from build123d import *

# Parameters (mm, degrees)
SKETCH_1_W          = 9
SKETCH_1_H          = 6.5
EXTRUDE_1_DEPTH     = 815
SKETCH_2_R          = 1.750000006
CUT_EXTRUDE_1_DEPTH = 726.778225985
SKETCH_3_R          = 3.000000006
CUT_EXTRUDE_2_DEPTH = 3.5


with BuildPart() as part:
    # 草图1 → 凸台-拉伸1 (new body)
    with BuildSketch(Plane.XY.offset(-89.264832522)):
        Rectangle(SKETCH_1_W, SKETCH_1_H)
    extrude(amount=EXTRUDE_1_DEPTH)

    # 草图2 → 切除-拉伸1 (cut, through all)
    with BuildSketch(Plane(origin=(0, 3.25, 0), x_dir=(1, 0, 0), z_dir=(0, 1, 0))):
        with Locations(Location((0, 81.764832522, 0), (0, 0, 270))):
            Circle(SKETCH_2_R)
        with Locations(Location((0, 61.764832522, 0), (0, 0, 270))):
            Circle(SKETCH_2_R)
        with Locations(Location((0, 41.764832522, 0), (0, 0, 270))):
            Circle(SKETCH_2_R)
        with Locations(Location((0, 21.764832522, 0), (0, 0, 270))):
            Circle(SKETCH_2_R)
        with Locations(Location((0, 1.764832522, 0), (0, 0, 270))):
            Circle(SKETCH_2_R)
        with Locations(Location((0, -18.235167478, 0), (0, 0, 270))):
            Circle(SKETCH_2_R)
        with Locations(Location((0, -38.235167478, 0), (0, 0, 270))):
            Circle(SKETCH_2_R)
        with Locations(Location((0, -58.235167478, 0), (0, 0, 270))):
            Circle(SKETCH_2_R)
        with Locations(Location((0, -78.235167478, 0), (0, 0, 270))):
            Circle(SKETCH_2_R)
        with Locations(Location((0, -98.235167478, 0), (0, 0, 270))):
            Circle(SKETCH_2_R)
        with Locations(Location((0, -118.235167478, 0), (0, 0, 270))):
            Circle(SKETCH_2_R)
        with Locations(Location((0, -138.235167478, 0), (0, 0, 270))):
            Circle(SKETCH_2_R)
        with Locations(Location((0, -158.235167478, 0), (0, 0, 270))):
            Circle(SKETCH_2_R)
        with Locations(Location((0, -178.235167478, 0), (0, 0, 270))):
            Circle(SKETCH_2_R)
        with Locations(Location((0, -198.235167478, 0), (0, 0, 270))):
            Circle(SKETCH_2_R)
        with Locations(Location((0, -218.235167478, 0), (0, 0, 270))):
            Circle(SKETCH_2_R)
        with Locations(Location((0, -238.235167478, 0), (0, 0, 270))):
            Circle(SKETCH_2_R)
        with Locations(Location((0, -258.235167478, 0), (0, 0, 270))):
            Circle(SKETCH_2_R)
        with Locations(Location((0, -278.235167478, 0), (0, 0, 270))):
            Circle(SKETCH_2_R)
        with Locations(Location((0, -298.235167478, 0), (0, 0, 270))):
            Circle(SKETCH_2_R)
        with Locations(Location((0, -318.235167478, 0), (0, 0, 270))):
            Circle(SKETCH_2_R)
        with Locations(Location((0, -338.235167478, 0), (0, 0, 270))):
            Circle(SKETCH_2_R)
        with Locations(Location((0, -358.235167478, 0), (0, 0, 270))):
            Circle(SKETCH_2_R)
        with Locations(Location((0, -378.235167478, 0), (0, 0, 270))):
            Circle(SKETCH_2_R)
        with Locations(Location((0, -398.235167478, 0), (0, 0, 270))):
            Circle(SKETCH_2_R)
        with Locations(Location((0, -418.235167478, 0), (0, 0, 270))):
            Circle(SKETCH_2_R)
        with Locations(Location((0, -438.235167478, 0), (0, 0, 270))):
            Circle(SKETCH_2_R)
        with Locations(Location((0, -458.235167478, 0), (0, 0, 270))):
            Circle(SKETCH_2_R)
        with Locations(Location((0, -478.235167478, 0), (0, 0, 270))):
            Circle(SKETCH_2_R)
        with Locations(Location((0, -498.235167478, 0), (0, 0, 270))):
            Circle(SKETCH_2_R)
        with Locations(Location((0, -518.235167478, 0), (0, 0, 270))):
            Circle(SKETCH_2_R)
        with Locations(Location((0, -538.235167478, 0), (0, 0, 270))):
            Circle(SKETCH_2_R)
        with Locations(Location((0, -558.235167478, 0), (0, 0, 270))):
            Circle(SKETCH_2_R)
        with Locations(Location((0, -578.235167478, 0), (0, 0, 270))):
            Circle(SKETCH_2_R)
        with Locations(Location((0, -598.235167478, 0), (0, 0, 270))):
            Circle(SKETCH_2_R)
        with Locations(Location((0, -618.235167478, 0), (0, 0, 270))):
            Circle(SKETCH_2_R)
        with Locations(Location((0, -638.235167478, 0), (0, 0, 270))):
            Circle(SKETCH_2_R)
        with Locations(Location((0, -658.235167478, 0), (0, 0, 270))):
            Circle(SKETCH_2_R)
        with Locations(Location((0, -678.235167478, 0), (0, 0, 270))):
            Circle(SKETCH_2_R)
        with Locations(Location((0, -698.235167478, 0), (0, 0, 270))):
            Circle(SKETCH_2_R)
        with Locations(Location((0, -718.235167478, 0), (0, 0, 270))):
            Circle(SKETCH_2_R)
        with Locations((0, -738.235167478)):
            Circle(SKETCH_2_R)
        with Locations((0, -758.235167478)):
            Circle(SKETCH_2_R)
        with Locations((0, -778.235167478)):
            Circle(SKETCH_2_R)
        with Locations((0, -798.235167478)):
            Circle(SKETCH_2_R)
        with Locations((0, -818.235167478)):
            Circle(SKETCH_2_R)
        with Locations((0, -838.235167478)):
            Circle(SKETCH_2_R)
        with Locations((0, -858.235167478)):
            Circle(SKETCH_2_R)
        with Locations((0, -878.235167478)):
            Circle(SKETCH_2_R)
        with Locations((0, -898.235167478)):
            Circle(SKETCH_2_R)
        with Locations((0, -918.235167478)):
            Circle(SKETCH_2_R)
        with Locations((0, -938.235167478)):
            Circle(SKETCH_2_R)
        with Locations((0, -958.235167478)):
            Circle(SKETCH_2_R)
        with Locations((0, -978.235167478)):
            Circle(SKETCH_2_R)
        with Locations((0, -998.235167478)):
            Circle(SKETCH_2_R)
        with Locations((0, -1018.235167478)):
            Circle(SKETCH_2_R)
        with Locations((0, -1038.235167478)):
            Circle(SKETCH_2_R)
        with Locations((0, -1058.235167478)):
            Circle(SKETCH_2_R)
        with Locations((0, -1078.235167478)):
            Circle(SKETCH_2_R)
        with Locations((0, -1098.235167478)):
            Circle(SKETCH_2_R)
    extrude(amount=-CUT_EXTRUDE_1_DEPTH, mode=Mode.SUBTRACT)

    # 草图3 → 切除-拉伸2 (cut)
    with BuildSketch(Plane(origin=(0, 3.25, 0), x_dir=(1, 0, 0), z_dir=(0, 1, 0))):
        with Locations(Location((0, 81.764832522, 0), (0, 0, 270))):
            Circle(SKETCH_3_R)
        with Locations(Location((0, 61.764832522, 0), (0, 0, 270))):
            Circle(SKETCH_3_R)
        with Locations(Location((0, 41.764832522, 0), (0, 0, 270))):
            Circle(SKETCH_3_R)
        with Locations(Location((0, 21.764832522, 0), (0, 0, 270))):
            Circle(SKETCH_3_R)
        with Locations(Location((0, 1.764832522, 0), (0, 0, 270))):
            Circle(SKETCH_3_R)
        with Locations(Location((0, -18.235167478, 0), (0, 0, 270))):
            Circle(SKETCH_3_R)
        with Locations(Location((0, -38.235167478, 0), (0, 0, 270))):
            Circle(SKETCH_3_R)
        with Locations(Location((0, -58.235167478, 0), (0, 0, 270))):
            Circle(SKETCH_3_R)
        with Locations(Location((0, -78.235167478, 0), (0, 0, 270))):
            Circle(SKETCH_3_R)
        with Locations(Location((0, -98.235167478, 0), (0, 0, 270))):
            Circle(SKETCH_3_R)
        with Locations(Location((0, -118.235167478, 0), (0, 0, 270))):
            Circle(SKETCH_3_R)
        with Locations(Location((0, -138.235167478, 0), (0, 0, 270))):
            Circle(SKETCH_3_R)
        with Locations(Location((0, -158.235167478, 0), (0, 0, 270))):
            Circle(SKETCH_3_R)
        with Locations(Location((0, -178.235167478, 0), (0, 0, 270))):
            Circle(SKETCH_3_R)
        with Locations(Location((0, -198.235167478, 0), (0, 0, 270))):
            Circle(SKETCH_3_R)
        with Locations(Location((0, -218.235167478, 0), (0, 0, 270))):
            Circle(SKETCH_3_R)
        with Locations(Location((0, -238.235167478, 0), (0, 0, 270))):
            Circle(SKETCH_3_R)
        with Locations(Location((0, -258.235167478, 0), (0, 0, 270))):
            Circle(SKETCH_3_R)
        with Locations(Location((0, -278.235167478, 0), (0, 0, 270))):
            Circle(SKETCH_3_R)
        with Locations(Location((0, -298.235167478, 0), (0, 0, 270))):
            Circle(SKETCH_3_R)
        with Locations(Location((0, -318.235167478, 0), (0, 0, 270))):
            Circle(SKETCH_3_R)
        with Locations(Location((0, -338.235167478, 0), (0, 0, 270))):
            Circle(SKETCH_3_R)
        with Locations(Location((0, -358.235167478, 0), (0, 0, 270))):
            Circle(SKETCH_3_R)
        with Locations(Location((0, -378.235167478, 0), (0, 0, 270))):
            Circle(SKETCH_3_R)
        with Locations(Location((0, -398.235167478, 0), (0, 0, 270))):
            Circle(SKETCH_3_R)
        with Locations(Location((0, -418.235167478, 0), (0, 0, 270))):
            Circle(SKETCH_3_R)
        with Locations(Location((0, -438.235167478, 0), (0, 0, 270))):
            Circle(SKETCH_3_R)
        with Locations(Location((0, -458.235167478, 0), (0, 0, 270))):
            Circle(SKETCH_3_R)
        with Locations(Location((0, -478.235167478, 0), (0, 0, 270))):
            Circle(SKETCH_3_R)
        with Locations(Location((0, -498.235167478, 0), (0, 0, 270))):
            Circle(SKETCH_3_R)
        with Locations(Location((0, -518.235167478, 0), (0, 0, 270))):
            Circle(SKETCH_3_R)
        with Locations(Location((0, -538.235167478, 0), (0, 0, 270))):
            Circle(SKETCH_3_R)
        with Locations(Location((0, -558.235167478, 0), (0, 0, 270))):
            Circle(SKETCH_3_R)
        with Locations(Location((0, -578.235167478, 0), (0, 0, 270))):
            Circle(SKETCH_3_R)
        with Locations(Location((0, -598.235167478, 0), (0, 0, 270))):
            Circle(SKETCH_3_R)
        with Locations(Location((0, -618.235167478, 0), (0, 0, 270))):
            Circle(SKETCH_3_R)
        with Locations(Location((0, -638.235167478, 0), (0, 0, 270))):
            Circle(SKETCH_3_R)
        with Locations(Location((0, -658.235167478, 0), (0, 0, 270))):
            Circle(SKETCH_3_R)
        with Locations(Location((0, -678.235167478, 0), (0, 0, 270))):
            Circle(SKETCH_3_R)
        with Locations(Location((0, -698.235167478, 0), (0, 0, 270))):
            Circle(SKETCH_3_R)
        with Locations(Location((0, -718.235167478, 0), (0, 0, 270))):
            Circle(SKETCH_3_R)
        with Locations((0, -738.235167478)):
            Circle(SKETCH_3_R)
        with Locations((0, -758.235167478)):
            Circle(SKETCH_3_R)
        with Locations((0, -778.235167478)):
            Circle(SKETCH_3_R)
        with Locations((0, -798.235167478)):
            Circle(SKETCH_3_R)
        with Locations((0, -818.235167478)):
            Circle(SKETCH_3_R)
        with Locations((0, -838.235167478)):
            Circle(SKETCH_3_R)
        with Locations((0, -858.235167478)):
            Circle(SKETCH_3_R)
        with Locations((0, -878.235167478)):
            Circle(SKETCH_3_R)
        with Locations((0, -898.235167478)):
            Circle(SKETCH_3_R)
        with Locations((0, -918.235167478)):
            Circle(SKETCH_3_R)
        with Locations((0, -938.235167478)):
            Circle(SKETCH_3_R)
        with Locations((0, -958.235167478)):
            Circle(SKETCH_3_R)
        with Locations((0, -978.235167478)):
            Circle(SKETCH_3_R)
        with Locations((0, -998.235167478)):
            Circle(SKETCH_3_R)
        with Locations((0, -1018.235167478)):
            Circle(SKETCH_3_R)
        with Locations((0, -1038.235167478)):
            Circle(SKETCH_3_R)
        with Locations((0, -1058.235167478)):
            Circle(SKETCH_3_R)
        with Locations((0, -1078.235167478)):
            Circle(SKETCH_3_R)
        with Locations((0, -1098.235167478)):
            Circle(SKETCH_3_R)
    extrude(amount=-CUT_EXTRUDE_2_DEPTH, mode=Mode.SUBTRACT)


solid = part.part
The model under review builds one solid part; all positions refer to its coordinate system, in mm. Coordinates: 2 decimals unless noted, no trailing zeros. Answer in a Markdown table with one row per item.
1. Clearance check with flat-ended pins moving along their axes: pin 1 Ø4.5 at (x, z) = (0, 178.24) entering from +Y; pin 2 Ø4.5 at (x, z) = (0, 98.24) entering from -Y; pin 3 Ø3 at (x, z) = (0, 38.24) entering from -Y. State where each tip first meets the part, or that it passes through.
Answers below:
| item | result |
|---|---|
| pin 1 | stops at y = -0.25 |
| pin 2 | stops at y = -3.25 |
| pin 3 | passes through |
2. Wall thickness on probe 1 along X at (y, z) = (-2.5, 558.5); probe 2 along Y at (x, z) = (-0.75, 616); probe 3 along X at (y, z) = (2.5, 297): over which ranges is each line inside the solid? List them lowest first. Write a range as [from, to].
Answers below:
| item | result |
|---|---|
| probe 1 | x = [-4.5, -1.73], [1.73, 4.5] |
| probe 2 | y = [-3.25, -0.25] |
| probe 3 | x = [-4.5, -2.73], [2.73, 4.5] |
3. We need section A-A, the plane x = 0. Give the number of separate pieces and of enclosed holes in the cut face, and give its area (3 significant figures).
Answers below:
| item | result |
|---|---|
| separate pieces | 42 |
| enclosed holes | 0 |
| area | 4,010 mm^2 |
